Autodesk Inventor part; units mm, degrees
ref_plane "Work Plane2" through (0, -3.175, 0) normal (0, -1, 0) x (1, 0, 0)
ref_plane "YZ Plane" through (0, 0, 0) normal (1, 0, 0) x (0, 1, 0)
ref_plane "XZ Plane" through (0, 0, 0) normal (0, 1, 0) x (-1, 0, 0)
sketch "Sketch1" plane through (0, 0, 0) normal (0, 1, 0) x (-1, 0, 0)
  line L0 (-301.6, 175.65) -> (-203.3004, 175.65)
  line L1 (-203.3004, 275.65) -> (-301.6, 275.65)
  line L2 (-301.6, 275.65) -> (-301.6, 175.65)
  line L3 (-301.6, 275.65) -> (-201.6, 275.65)
  line L4 (-201.6, 275.65) -> (-201.6, 175.65)
  line L5 (-201.6, 175.65) -> (-301.6, 175.65)
  line L6 (-301.6, 175.65) -> (-301.6, 275.65)
  line L7 (-301.6, 175.65) -> (-301.6, 275.65)
  line L8 (-301.6, 275.65) -> (-201.6, 275.65)
  line L9 (-201.6, 275.65) -> (-201.6, 75.65)
  line L10 (-301.6, 75.65) -> (-301.6, 275.65)
  line L11 (-301.6, 75.65) -> (-301.6, 275.65)
  line L12 (-152.1, 75.65) -> (-162.1, 75.65)
  line L13 (-157.1, 260.65) -> (-57.1, 260.65)
  line L14 (-52.1, 265.65) -> (-52.1, 265.65)
  line L15 (-57.1, 270.65) -> (-157.1, 270.65)
  circle A0 centre (-346.1, 265.65) radius 5
  arc A1 (-157.1, 270.65) -> (-157.1, 260.65) centre (-157.1, 265.65) ccw
  line L16 (-201.6, 75.65) -> (-157.1, 75.65)
  arc A2 (-152.1, 185.65) -> (-162.1, 185.65) centre (-157.1, 185.65) ccw
  line L17 (-162.1, 185.65) -> (-162.1, 85.65)
  line L18 (-152.1, 75.65) -> (-152.1, 185.65)
  line L19 (-157.1, 80.65) -> (-157.1, 80.65)
  arc A3 (-341.1, 185.65) -> (-351.1, 185.65) centre (-346.1, 185.65) ccw
  line L20 (-341.1, 85.65) -> (-341.1, 185.65)
  line L21 (-351.1, 185.65) -> (-351.1, 85.65)
  line L22 (-346.1, 80.65) -> (-346.1, 80.65)
  line L23 (-301.6, 275.65) -> (-201.6, 275.65)
  line L24 (-201.6, 275.65) -> (-201.6, 49.35)
  line L25 (-201.6, 49.35) -> (-301.6, 49.35)
  line L26 (-301.6, 49.35) -> (-301.6, 275.65)
  line L27 (-351.1, 85.65) -> (-351.1, 59.35)
  line L28 (-341.1, 59.35) -> (-341.1, 85.65)
  arc A4 (-351.1, 59.35) -> (-341.1, 59.35) centre (-346.1, 59.35) ccw
  line L29 (-152.1, 80.65) -> (-152.1, 64.35)
  line L30 (-162.1, 59.35) -> (-162.1, 85.65)
  arc A5 (-162.1, 59.35) -> (-157.1, 54.35) centre (-157.1, 59.35) ccw
  line L31 (-301.6, 49.35) -> (-75.3, 49.35)
  line L32 (-75.3, 49.35) -> (-75.3, 275.65)
  line L33 (-75.3, 275.65) -> (-201.6, 275.65)
  line L34 (-157.1, 54.35) -> (-30.8, 54.35)
  arc A6 (-30.8, 54.35) -> (-30.8, 64.35) centre (-30.8, 59.35) ccw
  line L35 (-30.8, 64.35) -> (-152.1, 64.35)
  line L36 (-57.1, 260.65) -> (-30.8, 260.65)
  line L37 (-57.1, 270.65) -> (-30.8, 270.65)
  arc A7 (-30.8, 260.65) -> (-30.8, 270.65) centre (-30.8, 265.65) ccw
  line L38 (-69.2464, 270.65) -> (-69.2464, 286.45)
  line L39 (2.2, 286.45) -> (-379.1, 286.45)
  line L40 (-52.1, 54.35) -> (-52.1, 38.55)
  line L41 (2.2, 38.55) -> (-379.1, 38.55)
  line L42 (-25.8, 59.35) -> (-4.8, 59.35)
  line L43 (2.2, 38.55) -> (2.2, 286.45)
  line L44 (-4.8, 99) -> (-4.8, 226)
  line L45 (-372.1, 99) -> (-372.1, 226)
  line L46 (-379.1, 38.55) -> (-379.1, 286.45)
  point P0 (-52.1, 270.65)
  point P1 (-52.1, 260.65)
  point P2 (-157.1, 85.65)
  point P3 (-157.1, 185.65)
  point P4 (-157.1, 85.65)
  point P5 (-162.1, 80.65)
  point P6 (0, 305)
  point P7 (-152.1, 75.65)
  dimension "d2" = 100
  dimension "d3" = 100
  dimension "d7" = 10
  dimension "d8" = 10
  dimension "d16" = 10
  dimension "d17" = 44.5
  dimension "d20" = 10
  dimension "d21" = 10
  dimension "d22" = 10
  dimension "d70" = 226.3
  dimension "d72" = 10
  dimension "d73" = 10
  dimension "d180" = 226.3
  dimension "d224" = 15.8
  dimension "d227" = 15.8
  dimension "d229" = 21
  dimension "d233" = 127
  dimension "d235" = 127
extrude "Extrusion1" add sketch "Sketch1" along normal blind 3.175 contours L2 L1 L3 L4 L5 L0 | L10 L26 L25 L31 L32 L34 L40 L41 L46 L39 L38 L15 L33 L3 L1 L2 | L0 L5 L9 L24 L25 L26 L10 | L4 L33 L32 L15 A1 L13 L35 L29 L18 A2 L17 L30 L16 L9 | L16 L30 A5 L34 L32 L31 L24 | L38 L39 L43 L41 L40 L34 A6 L35 L32 L13 L36 A7 L37 L15
sketch "Sketch2" plane through (0, 0, 0) normal (0, -1, 0) x (1, 0, 0)
  line L0 (346.1, 80.65) -> (346.1, 80.65)
  line L1 (353.1, 85.65) -> (353.1, 190.65)
  line L2 (339.1, 190.65) -> (339.1, 85.65)
  line L3 (339.1, 85.65) -> (339.1, 54.35)
  line L4 (353.1, 54.35) -> (353.1, 85.65)
  circle A0 centre (346.1, 265.65) radius 7.25
  line L5 (57.1, 258.65) -> (162.1, 258.65)
  line L6 (162.1, 272.65) -> (57.1, 272.65)
  line L7 (57.1, 272.65) -> (25.8, 272.65)
  line L8 (25.8, 258.65) -> (57.1, 258.65)
  line L9 (25.8, 59.35) -> (25.8, 59.35)
  line L10 (157.1, 190.65) -> (157.1, 190.65)
  line L11 (152.1, 185.65) -> (152.1, 64.35)
  line L12 (25.8, 52.35) -> (157.1, 52.35)
  arc A1 (157.1, 52.35) -> (164.1, 59.35) centre (157.1, 59.35) ccw
  line L13 (164.1, 59.35) -> (164.1, 190.65)
  line L14 (150.1, 190.65) -> (150.1, 73.35)
  line L15 (143.1, 66.35) -> (25.8, 66.35)
  arc A2 (143.1, 66.35) -> (150.1, 73.35) centre (143.1, 73.35) ccw
  line L16 (346.1, 185.65) -> (346.1, 190.65)
  arc A3 (353.1, 190.65) -> (339.1, 190.65) centre (346.1, 190.65) ccw
  arc A4 (339.1, 54.35) -> (353.1, 54.35) centre (346.1, 54.35) ccw
  arc A5 (164.1, 190.65) -> (150.1, 190.65) centre (157.1, 190.65) ccw
  arc A6 (25.8, 66.35) -> (25.8, 52.35) centre (25.8, 59.35) ccw
  arc A7 (30.8, 270.65) -> (30.8, 260.65) centre (30.8, 265.65) ccw
  arc A8 (25.8, 272.65) -> (25.8, 258.65) centre (25.8, 265.65) ccw
  arc A9 (162.1, 258.65) -> (162.1, 272.65) centre (162.1, 265.65) ccw
  point P0 (0, 305)
  point P1 (52.1, 260.65)
  dimension "d209" = 7
  dimension "d212" = 5
  dimension "d213" = 14
  dimension "d215" = 14
  dimension "d217" = 14
  dimension "d219" = 14
  dimension "d221" = 14
  dimension "d223" = 14
extrude "Extrusion2" cut sketch "Sketch2" against normal blind 2
sketch "Sketch4" plane through (0, 0, 0) normal (0, -1, 0) x (1, 0, 0)
  line L0 (339.1, 54.35) -> (339.1, 190.65)
  line L1 (353.1, 190.65) -> (353.1, 54.35)
  line L2 (150.1, 73.35) -> (150.1, 190.65)
  line L3 (164.1, 190.65) -> (164.1, 59.35)
  arc A0 (157.1, 52.35) -> (164.1, 59.35) centre (157.1, 59.35) ccw
  line L4 (157.1, 52.35) -> (25.8, 52.35)
  arc A1 (143.1, 66.35) -> (150.1, 73.35) centre (143.1, 73.35) ccw
  line L5 (25.8, 66.35) -> (143.1, 66.35)
  circle A2 centre (346.1, 265.65) radius 7.25
  line L6 (162.1, 258.65) -> (25.8, 258.65)
  line L7 (25.8, 272.65) -> (162.1, 272.65)
  arc A3 (339.1, 54.35) -> (353.1, 54.35) centre (346.1, 54.35) ccw
  arc A4 (353.1, 190.65) -> (339.1, 190.65) centre (346.1, 190.65) ccw
  arc A5 (164.1, 190.65) -> (150.1, 190.65) centre (157.1, 190.65) ccw
  arc A6 (25.8, 66.35) -> (25.8, 52.35) centre (25.8, 59.35) ccw
  arc A7 (162.1, 258.65) -> (162.1, 272.65) centre (162.1, 265.65) ccw
  arc A8 (25.8, 272.65) -> (25.8, 258.65) centre (25.8, 265.65) ccw
  line L8 (-2.2, 286.45) -> (379.1, 286.45)
  line L9 (379.1, 38.55) -> (-2.2, 38.55)
  line L10 (-2.2, 38.55) -> (-2.2, 286.45)
  line L11 (379.1, 286.45) -> (379.1, 38.55)
  point P0 (353.1, 59.35)
  point P1 (339.1, 59.35)
  point P2 (339.1, 185.65)
  point P3 (353.1, 185.65)
  point P4 (150.1, 185.65)
  point P5 (164.1, 185.65)
  point P6 (30.8, 52.35)
  point P7 (30.8, 66.35)
  point P8 (157.1, 258.65)
  point P9 (30.8, 258.65)
  point P10 (157.1, 272.65)
  point P11 (30.8, 272.65)
extrude "Extrusion4" add sketch "Sketch4" along normal blind 3.175
fillet "Fillet2" radius 20 4 edges at (-2.2, 0, 286.45) (379.1, 0, 286.45) (379.1, 0, 38.55) (-2.2, 0, 38.55)
ref_plane "Work Plane2" through (0, -3.175, 0) normal (0, -1, 0) x (1, 0, 0)
sketch "Sketch6" plane through (0, -3.175, 0) normal (0, -1, 0) x (1, 0, 0)
  line L0 (4.8, 99) -> (4.8, 226)
  line L1 (372.1, 99) -> (372.1, 226)
  point P0 (0, 0)
hole "Hole1" at (4.8, -3.175, 226) at (4.8, -3.175, 99) at (372.1, -3.175, 226) at (372.1, -3.175, 99) direction (0, 1, 0) diameter 8 end through all counterbore diameter 12 counterbore depth 5.175
properties part number "PlateAxial" material "Aluminum, Anodized Silver"
The model under review builds one solid part; all positions refer to its coordinate system, in mm. A direction names the side the tool comes from. Round coordinates to 2 decimals unless told otherwise and drop trailing zeros. Loops run counter-clockwise (first coordinate to the right, second up) from the corner with the lowest first, then second, coordinate; pieces in that order, holes last. Notation, with made-up numbers: M 44.25,46 L 90.25,46 A14 cw 90.25,66 Z; hole C 25.5,84 d11. An arc over 180 degrees is marked long. Answer as a JSON object with one key per item and string values.
Item 1: Tool access review of faces 4 (the face through (348, 2, 271)), 5 (the face through (375.649, 2.596, 97.154)): name each direction out of +Z, -Z, +X, -X, +Y, -Y from which nothing blocks a thin tool from reaching the whole face with its end or side.
Check sheet entries:
{"face 4": "-Y", "face 5": "+Y, -Y"}
Item 2: We need section A-A, the plane z = 109.5. State the section outline as (x, y) points (3 decimals).
Check sheet entries:
{"outline": "M -2.2,-3.175 L 150.1,-3.175 L 150.1,2 L 152.1,2 L 152.1,3.175 L -2.2,3.175 Z; M 162.1,2 L 164.1,2 L 164.1,-3.175 L 339.1,-3.175 L 339.1,2 L 341.1,2 L 341.1,3.175 L 162.1,3.175 Z; M 351.1,2 L 353.1,2 L 353.1,-3.175 L 379.1,-3.175 L 379.1,3.175 L 351.1,3.175 Z"}
Item 3: We need section C-C, the plane y = 1. State how many separate pieces and enclosed holes the cut face has, and give its area (3 significant figures).
Check sheet entries:
{"separate pieces": "1", "enclosed holes": "8", "area": "85,600 mm2"}
Item 4: For line 1 along X through (y, z) = (0.25, 77); line 2 along Z through (x, y) = (61, 0.5); line 3 along Z through (x, y) = (346.1, 2.7), list the stretches that pass through material, from the lowest coordinate up.
Check sheet entries:
{"line 1": "-2.2 to 150.1, 164.1 to 339.1, 353.1 to 379.1", "line 2": "38.55 to 52.35, 66.35 to 258.65, 272.65 to 286.45", "line 3": "38.55 to 54.35, 190.65 to 260.65, 270.65 to 286.45"}
Item 5: We need section B-B, the plane x = 346.1. State the section outline as (y, z) points (3 decimals).
Check sheet entries:
{"outline": "M -3.175,38.55 L 3.175,38.55 L 3.175,54.35 L 2,54.35 L 2,47.35 L -3.175,47.35 Z; M -3.175,197.65 L 2,197.65 L 2,190.65 L 3.175,190.65 L 3.175,260.65 L 2,260.65 L 2,258.4 L -3.175,258.4 Z; M -3.175,272.9 L 2,272.9 L 2,270.65 L 3.175,270.65 L 3.175,286.45 L -3.175,286.45 Z"}
Item 6: The part is to be moulded in two halves that separate along Z. For faces 1 (the face through (191, 3.175, 164)), 2 (the face through (373.086, 0.044, 280.747)), 3 (the face through (345.95, -0.55, 197.65)), say which applies: +Z half, -Z half, draft (parallel to the pull), parting line (faces both ways), or undercut.
Check sheet entries:
{"face 1": "draft", "face 2": "+Z half", "face 3": "undercut"}
Item 7: Clearance check with a flat-ended pin moving along its axis: P1, Ø6, axis at x = 4.5, z = 227, coming from the -Y side. State where the tip first meets the part, or that it passes through.
Check sheet entries:
{"P1": "y = 2"}
